Source: CAD feature listing. Evaluate the final solid. Frame: model axes, mm. Give positions to 0.01 mm unless a question says otherwise; leave off trailing zeros. Loops run counter-clockwise (first coordinate to the right, second up) from the corner with the lowest first, then second, coordinate; pieces in that order, holes last.
Autodesk Inventor part; units mm, degrees
ref_plane "Work Plane1" through (15, 0, 0) normal (1, 0, 0) x (0, 0, -1)
ref_plane "YZ Plane" through (0, 0, 0) normal (1, 0, 0) x (0, 1, 0)
ref_plane "XZ Plane" through (0, 0, 0) normal (0, 1, 0) x (-1, 0, 0)
sketch "Sketch1" plane through (0, 0, 0) normal (0, 0, 1) x (1, 0, 0)
  line L0 (0, 0) -> (30, 0)
  line L1 (30, 0) -> (30, 50)
  line L2 (30, 50) -> (0, 50)
  line L3 (0, 50) -> (0, 0)
  dimension "d0" = 30
  dimension "d1" = 50
extrude "Extrusion1" add sketch "Sketch1" along normal blind 3
sketch "Sketch2" plane through (30, 0, 0) normal (1, 0, 0) x (0, 0, -1)
  line L0 (-1.5, 30) -> (-1.5, 20) construction
  line L1 (-3, 0) -> (-3, 50)
  line L2 (-2.5, 29) -> (-2.5, 21)
  line L3 (-0.5, 21) -> (-0.5, 29)
  arc A0 (-0.5, 29) -> (-2.5, 29) centre (-1.5, 29) ccw
  arc A1 (-2.5, 21) -> (-0.5, 21) centre (-1.5, 21) ccw
  line L4 (0, 0) -> (0, 50)
  point P0 (-1.5, 25)
  point P1 (0, 25)
  dimension "d12" = 25
  dimension "d13" = 1
  dimension "d14" = 10
  dimension "d15" = 1.5
extrude "Extrusion2" cut sketch "Sketch2" against normal blind 3.7
ref_plane "Work Plane1" through (15, 0, 0) normal (1, 0, 0) x (0, 0, -1)
mirror "Mirror1" about plane through (15, 0, 0) normal (1, 0, 0) of "Extrusion2"
properties part number "motor box 2"
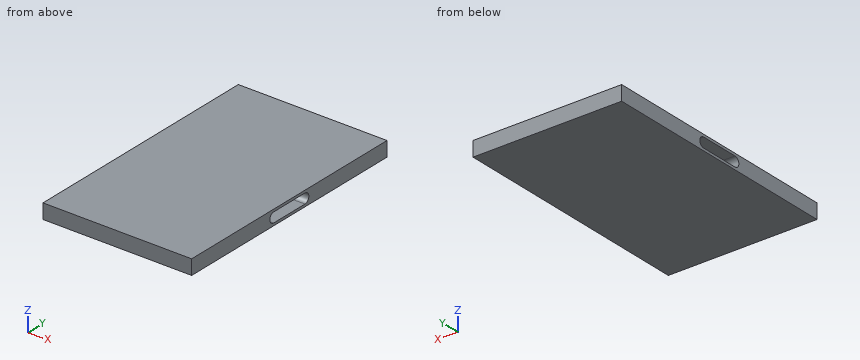
1) Contact query for flat-ended pins moving along their axis: P1, Ø4, axis at x = 28, y = 26, coming from the -Z side; P2, Ø1, axis at y = 27.5, z = 1.5, coming from the +X side. Output: stop coordinate, or through.
Checks:
P1: stops at z = 0
P2: stops at x = 26.3
2) Ray query, probe 1 along Z at (x, y) = (1.5, 25); probe 2 along X at (y, z) = (26, 1.9). Return the intervals inside material, ascending.
Checks:
probe 1: z = 0 to 0.5, 2.5 to 3
probe 2: x = 3.7 to 26.3
3) Cut plane B-B (z = 1.5). Return loops of the section in (x, y), and give its area (3 significant figures).
Checks:
outline: (0, 0) - (30, 0) - (30, 20) - (26.3, 20) - (26.3, 30) - (30, 30) - (30, 50) - (0, 50) - (0, 30) - (3.7, 30) - (3.7, 20) - (0, 20) - close
area: 1,430 mm2
4) Cut plane A-A (x = 27.75). Return loops of the section in (y, z).
Checks:
outline: (0, 0) - (50, 0) - (50, 3) - (0, 3) - close; hole (21, 0.5) - (29, 0.5) arc R1 ccw to (29, 2.5) - (21, 2.5) arc R1 ccw to start
